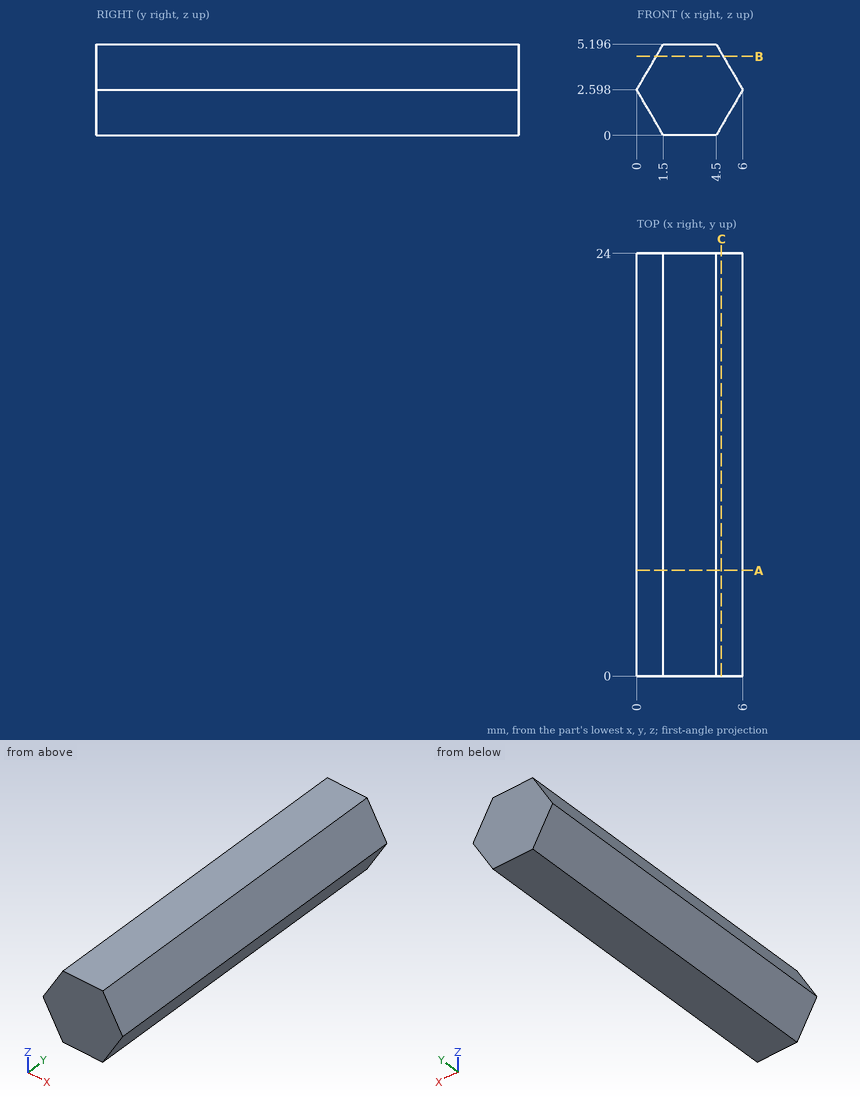
Here's the drawing with two shaded views (mm, measured from the low corner). I have some questions. Give positions to 0.01 mm unless a question says otherwise; leave off trailing zeros. Loops run counter-clockwise (first coordinate to the right, second up) from the corner with the lowest first, then second, coordinate; pieces in that order, holes last. Notation, with made-up numbers: (15, 66) - (35, 66) arc R22 ccw to (35, 85) - close; hole circle Ø10 at (5.25, 83). An arc over 180 degrees is marked (long way). Return JSON: item names as keys, results as strings.
1. If I drill on line 1 (X direction, y = 22, z = 2.4) (1 decimal); line 2 (X direction, y = 11, z = 1.2); line 3 (Z direction, x = 1, y = 14.75) (1 decimal), over which ranges is the centre line in solid material (lowest first)?
Output values:
{"line 1": "x = 0.1 to 5.9", "line 2": "x = 0.81 to 5.19", "line 3": "z = 0.9 to 4.3"}
2. I'm going to push a flat-ended pin straight in: pin 1 Ø1.5 at (y, z) = (16.5, 4) entering from +X. Where does the tip first touch, or does it pass through?
Output values:
{"pin 1": "stops at x = 5.62"}
3. I want a section at B-B on z = 4.5. Please give me the cut outline in (x, y), and give its area (3 significant figures).
Output values:
{"outline": "(1.1, 0) - (4.9, 0) - (4.9, 24) - (1.1, 24) - close", "area": "91.3 mm²"}
4. I want a section at A-A on y = 6. Please give me the cut outline in (x, z), and give its area (3 significant figures).
Output values:
{"outline": "(0, 2.6) - (1.5, 0) - (4.5, 0) - (6, 2.6) - (4.5, 5.2) - (1.5, 5.2) - close", "area": "23.4 mm²"}
5. I want a section at C-C on x = 4.8. Please give me the cut outline in (y, z).
Output values:
{"outline": "(0, 0.52) - (24, 0.52) - (24, 4.68) - (0, 4.68) - close"}
